Source: CAD feature listing. Evaluate the final solid. Frame: model axes, mm. A direction names the side the tool comes from. Round coordinates to 2 decimals unless told otherwise and drop trailing zeros. Order: outer loops, then holes, each group sorted by start corner. A loop starts at its lowest first (then second) coordinate and runs counter-clockwise, first axis right, second up. Notation, with made-up numbers: (49, 16) -> (63, 16) arc R29 ccw to (63, 55) -> close; hole circle Ø6 at (38.25, -36.5). An arc over 180 degrees is marked (long way). Use a Markdown table: item, result. Add a question column.
```python
from build123d import *

# Parameters (mm, degrees)
SKETCH1_W           = 80
SKETCH1_H           = 45
BOSS_EXTRUDE1_DEPTH = 5
SKETCH2_R           = 2.5
SKETCH2_W           = 41
SKETCH2_H           = 21.3
CUT_EXTRUDE1_DEPTH  = 10
CUT_EXTRUDE2_DEPTH  = 10
FILLET1_R           = 10


with BuildPart() as part:
    # Sketch1 → Boss-Extrude1 (new body)
    with BuildSketch(Plane.XY):
        Rectangle(SKETCH1_W, SKETCH1_H)
    extrude(amount=BOSS_EXTRUDE1_DEPTH)

    # Sketch2 → Cut-Extrude1 (cut)
    with BuildSketch(Plane.XY.offset(5)):
        with Locations((-24.25, -2.1)):
            Circle(SKETCH2_R)
        with Locations((-24.25, 7.72372371)):
            Circle(SKETCH2_R)
        with Locations((24.25, 7.72372371)):
            Circle(SKETCH2_R)
        with Locations((24.25, -2.1)):
            Circle(SKETCH2_R)
        with Locations((0, 2.5)):
            Rectangle(SKETCH2_W, SKETCH2_H)
    extrude(amount=-CUT_EXTRUDE1_DEPTH, mode=Mode.SUBTRACT)

    # Sketch3 → Cut-Extrude2 (cut)
    with BuildSketch(Plane.XY.offset(5)):
        Polygon((-36, -16.5), (-36, -22.5), (-34, -22.5), (-34, -10.5), (-36, -10.5), (-36, -12.5), (-37.5, -12.5), (-37.5, -16.5), align=None)
        Polygon((-34, -10.5), (-34, -22.5), (-32, -22.5), (-32, -16.5), (-30.5, -16.5), (-30.5, -12.5), (-32, -12.5), (-32, -10.5), align=None)
        Polygon((32, -16.5), (32, -22.5), (34, -22.5), (34, -10.5), (32, -10.5), (32, -12.5), (30.5, -12.5), (30.5, -16.5), align=None)
        Polygon((34, -10.5), (34, -22.5), (36, -22.5), (36, -16.5), (37.5, -16.5), (37.5, -12.5), (36, -12.5), (36, -10.5), align=None)
    extrude(amount=-CUT_EXTRUDE2_DEPTH, mode=Mode.SUBTRACT)

    # Fillet1
    fillet1_edges = [part.edges().sort_by_distance(p)[0] for p in [
        (-40, 22.5, 2.5),
        (40, 22.5, 2.5),
    ]]
    fillet(fillet1_edges, radius=FILLET1_R)


solid = part.part
```
1) Line query: probe 1 along Y at (x, z) = (24.25, 3.7); probe 2 along X at (y, z) = (-12, 2.9); probe 3 along X at (y, z) = (8, 1.45). Output: solid intervals per line, ascending. Write a range as from..to.
2) Section D-D on z = 4.15. Count the separate pieces of the cut face and the enclosed holes in it, then the cut area to 3 significant figures.
3) Section A-A on x = -19. Output: boundary loops of the cut face in (y, z).
4) Section B-B on y = -2.1. Output: boundary loops of the cut face in (x, z), then the cut area to 3 significant figures.
5) Draft query along X for faces 1 (the flat face through (0, 22.5, 2)), 2 (the cylindrical face through (21.752, -1.99, 2.535)), 3 (the cylindrical face through (-26.748, -1.99, 2.535)). Return one class per face: pulls with the +X half, pulls with the -X half, needs draft (parallel to the pull), parting line crosses it, or undercut.
6) Section C-C on x = 24.25. Output: boundary loops of the cut face in (y, z).
7) First-contact query: pin 1 Ø1.5 at (x, y) = (-20.5, 18) entering from -Z; pin 2 Ø1.2 at (x, z) = (37, 3) entering from +Y; pin 3 Ø1.2 at (x, z) = (-33, 3.5) entering from -Y; pin 4 Ø0.8 at (x, z) = (-31.5, 2.5) entering from +Y. Flat tips, straight axial feed; report the tip coordinate or a pass-through.
8) Reachability of faces 4 (the flat face through (-38, -22.5, 2)), 5 (the flat face through (-30.5, -15, 3)), 6 (the flat face through (-34, -10.5, 3)) from +Z, -Z, +X, -X, +Y, -Y: full face, straight path, thin tool, end or side. Return the list, or none.
Conclusion:
| question | item | result |
|---|---|---|
| 1 | probe 1 | y = -22.5..-4.6, 0.4..5.22, 10.22..22.5 |
| 1 | probe 2 | x = -40..-36, -32..32, 36..40 |
| 1 | probe 3 | x = -40..-26.73, -21.77..-20.5, 20.5..21.77, 26.73..40 |
| 2 | separate pieces | 1 |
| 2 | enclosed holes | 5 |
| 2 | area | 2,490 mm^2 |
| 3 | outline | (-22.5, 0) -> (-8.15, 0) -> (-8.15, 5) -> (-22.5, 5) -> close; (13.15, 0) -> (22.5, 0) -> (22.5, 5) -> (13.15, 5) -> close |
| 4 | outline | (-40, 0) -> (-26.75, 0) -> (-26.75, 5) -> (-40, 5) -> close; (-21.75, 0) -> (-20.5, 0) -> (-20.5, 5) -> (-21.75, 5) -> close; (20.5, 0) -> (21.75, 0) -> (21.75, 5) -> (20.5, 5) -> close; (26.75, 0) -> (40, 0) -> (40, 5) -> (26.75, 5) -> close |
| 4 | area | 145 mm^2 |
| 5 | face 1 | needs draft |
| 5 | face 2 | undercut |
| 5 | face 3 | undercut |
| 6 | outline | (-22.5, 0) -> (-4.6, 0) -> (-4.6, 5) -> (-22.5, 5) -> close; (0.4, 0) -> (5.22, 0) -> (5.22, 5) -> (0.4, 5) -> close; (10.22, 0) -> (22.5, 0) -> (22.5, 5) -> (10.22, 5) -> close |
| 7 | pin 1 | stops at z = 0 |
| 7 | pin 2 | stops at y = 20.18 |
| 7 | pin 3 | stops at y = -10.5 |
| 7 | pin 4 | stops at y = 22.44 |
| 8 | face 4 | +Z, -Z, +X, -X, -Y |
| 8 | face 5 | +Z, -Z |
| 8 | face 6 | +Z, -Z, -Y |
